Work out the finished part from the listing and answer in its coordinate system (mm). Round coordinates to 2 decimals unless told otherwise and drop trailing zeros. Order: outer loops, then holes, each group sorted by start corner. A loop starts at its lowest first (then second) coordinate and runs counter-clockwise, first axis right, second up. Notation, with made-up numbers: (84.5, 5.5) -> (118.5, 5.5) arc R20 cw to (118.5, 14.5) -> close; hole circle Ø11 at (42, 42.25). An arc over 180 degrees is marked (long way). Use a Markdown table: item, result. Add a question column.
Item 1: A cutting plane is placed at D-D, the plane z = 17.5. Determine the outline of the cut face in (x, y).
Item 2: Find the intervals of material crossed by L1, parallel to X at y = 5, z = 31.75 (3 decimals); L2, parallel to X at y = -5, z = -31, in increasing order. Write a range as [from, to].
Item 3: For a pull along Y with two mould halves and no side action, classify faces 1 (the cylindrical face through (3.84, -1.93, -21.57)), 2 (the flat face through (0, -6.35, 1)), 3 (the flat face through (6.35, 0, 1)) as +Y half, -Y half, draft (parallel to the pull), parting line (faces both ways), or undercut.
Item 4: A cutting plane is placed at A-A, the plane x = 5. Determine the outline of the cut face in (y, z) (3 decimals).
Item 5: A cutting plane is placed at C-C, the plane z = -19.05. Determine the outline of the cut face in (x, y) (3 decimals), plus the area to 3 significant figures.
from build123d import *

# Parameters (mm, degrees)
SKETCH1_W           = 12.7
SKETCH1_H           = 12.7
BOSS_EXTRUDE1_DEPTH = 38.1
SKETCH2_R           = 3.175
CUT_EXTRUDE1_DEPTH  = 41.659838908
SKETCH4_R           = 3.175
CUT_EXTRUDE2_DEPTH  = 41.659838908


with BuildPart() as part:
    # Sketch1 → Boss-Extrude1 (new, symmetric)
    with BuildSketch(Plane.XY):
        Rectangle(SKETCH1_W, SKETCH1_H)
    extrude(amount=BOSS_EXTRUDE1_DEPTH, both=True)

    # Sketch2 → Cut-Extrude1 (cut, through all)
    with BuildSketch(Plane(origin=(0, 6.35, 0), x_dir=(1, 0, 0), z_dir=(0, 1, 0))):
        with Locations(Location((0, 31.75, 0), (0, 0, 270))):
            Circle(SKETCH2_R)
        with Locations(Location((0, 19.05, 0), (0, 0, 270))):
            Circle(SKETCH2_R)
        with Locations(Location((0, 6.35, 0), (0, 0, 270))):
            Circle(SKETCH2_R)
        with Locations(Location((0, -6.35, 0), (0, 0, 270))):
            Circle(SKETCH2_R)
        with Locations(Location((0, -19.05, 0), (0, 0, 270))):
            Circle(SKETCH2_R)
        with Locations(Location((0, -31.75, 0), (0, 0, 270))):
            Circle(SKETCH2_R)
    extrude(amount=-CUT_EXTRUDE1_DEPTH, mode=Mode.SUBTRACT)

    # Sketch4 → Cut-Extrude2 (cut, through all)
    with BuildSketch(Plane.ZY.offset(6.35)):
        with Locations((31.75, 0)):
            Circle(SKETCH4_R)
        with Locations((19.05, 0)):
            Circle(SKETCH4_R)
        with Locations((6.35, 0)):
            Circle(SKETCH4_R)
        with Locations((-6.35, 0)):
            Circle(SKETCH4_R)
        with Locations((-19.05, 0)):
            Circle(SKETCH4_R)
        with Locations((-31.75, 0)):
            Circle(SKETCH4_R)
    extrude(amount=-CUT_EXTRUDE2_DEPTH, mode=Mode.SUBTRACT)


solid = part.part
Reported:
| question | item | result |
|---|---|---|
| 1 | outline | (-6.35, -6.35) -> (-2.77, -6.35) -> (-2.77, -2.77) -> (-6.35, -2.77) -> close; (-6.35, 2.77) -> (-2.77, 2.77) -> (-2.77, 6.35) -> (-6.35, 6.35) -> close; (2.77, -6.35) -> (6.35, -6.35) -> (6.35, -2.77) -> (2.77, -2.77) -> close; (2.77, 2.77) -> (6.35, 2.77) -> (6.35, 6.35) -> (2.77, 6.35) -> close |
| 2 | L1 | [-6.35, -3.175], [3.175, 6.35] |
| 2 | L2 | [-6.35, -3.09], [3.09, 6.35] |
| 3 | face 1 | undercut |
| 3 | face 2 | -Y half |
| 3 | face 3 | draft |
| 4 | outline | (-6.35, -38.1) -> (6.35, -38.1) -> (6.35, 38.1) -> (-6.35, 38.1) -> close; hole circle Ø6.35 at (0, -31.75); hole circle Ø6.35 at (0, -19.05); hole circle Ø6.35 at (0, -6.35); hole circle Ø6.35 at (0, 6.35); hole circle Ø6.35 at (0, 19.05); hole circle Ø6.35 at (0, 31.75) |
| 5 | outline | (-6.35, -6.35) -> (-3.175, -6.35) -> (-3.175, -3.175) -> (-6.35, -3.175) -> close; (-6.35, 3.175) -> (-3.175, 3.175) -> (-3.175, 6.35) -> (-6.35, 6.35) -> close; (3.175, -6.35) -> (6.35, -6.35) -> (6.35, -3.175) -> (3.175, -3.175) -> close; (3.175, 3.175) -> (6.35, 3.175) -> (6.35, 6.35) -> (3.175, 6.35) -> close |
| 5 | area | 40.3 mm² |
